from build123d import *

# Parameters (mm, degrees)
SKETCH_W        = 15.1
SKETCH_H        = 9
PAD_DEPTH       = 14.5
SKETCH001_W     = 13.1
SKETCH001_H     = 7
POCKET_DEPTH    = 13.5
SKETCH002_R     = 3.125
POCKET001_DEPTH = 5
POCKET002_DEPTH = 15.101


with BuildPart() as part:
    # Sketch → Pad (new body)
    with BuildSketch(Plane.XY):
        Rectangle(SKETCH_W, SKETCH_H)
    extrude(amount=PAD_DEPTH)

    # Sketch001 (on Face6 of Pad) → Pocket (cut)
    with BuildSketch(Plane.XY.offset(14.5)):
        Rectangle(SKETCH001_W, SKETCH001_H)
    extrude(amount=-POCKET_DEPTH, mode=Mode.SUBTRACT)

    # Sketch002 (on Face4 of Pocket) → Pocket001 (cut)
    with BuildSketch(Plane(origin=(0, 0, 0), x_dir=(1, 0, 0), z_dir=(0, 0, -1))):
        Circle(SKETCH002_R)
    extrude(amount=-POCKET001_DEPTH, mode=Mode.SUBTRACT)

    # Sketch003 (on Face2 of Pocket001) → Pocket002 (cut, through all)
    with BuildSketch(Plane(origin=(-7.55, 0, 0), x_dir=(0, -1, 0), z_dir=(-1, 0, 0))):
        with BuildLine():
            Line((-2.549494, 14.5), (2.549494, 14.5))
            Line((2.549494, 14.5), (2.549494, 11.50906))
            ThreePointArc((1.549494, 10.50906), (2.256601, 10.801953), (2.549494, 11.50906))
            Line((1.549494, 10.50906), (-1.549494, 10.50906))
            ThreePointArc((-2.549494, 11.50906), (-2.256601, 10.801953), (-1.549494, 10.50906))
            Line((-2.549494, 11.50906), (-2.549494, 14.5))
        make_face()
    extrude(amount=-POCKET002_DEPTH, mode=Mode.SUBTRACT)


solid = part.part
Geometry check sheet. Reference: the model listing, model coordinates, mm. A direction names the side the tool comes from. Coordinates: 2 decimals unless noted, no trailing zeros. Loops run counter-clockwise (first coordinate to the right, second up) from the corner with the lowest first, then second, coordinate; pieces in that order, holes last. Notation, with made-up numbers: (66.5, 70.25) - (99.5, 70.25) arc R24 ccw to (99.5, 84.25) - close; hole circle Ø4 at (-22, 69). An arc over 180 degrees is marked (long way). Use one line per item in the form item = value. Start each with the question number.
Item 1: Section check C-C, the plane z = 11.75. Enter the section's corners in (x, y).
Item 2: Thickness scan on probe 1 along Y at (x, z) = (0, 0.5) (3 decimals); probe 2 along Y at (x, z) = (-5, 12.5); probe 3 along X at (y, z) = (0.25, 4). Record the ranges inside material, lowest first.
Item 3: Section check D-D, the plane z = 7.75. Enter the section's corners in (x, y).
Item 4: Section check B-B, the plane y = 0. Enter the section's corners in (x, z) (3 decimals).
Item 5: Section check A-A, the plane x = 0. Enter the section's corners in (y, z) (3 decimals), and give its area (4 significant figures).
Item 6: Mould release check, pull along X, two halves, no side actions. Record for faces 1 (the face through (-6.55, 0, 6)), 2 (the face through (2.98, -0.94, 0.49)), 3 (the face through (7.55, 0, 7)), 4 (the face through (-3.5, 0.1, 0)): +X half, -X half, draft (parallel to the pull), parting line (faces both ways), or undercut.
Item 7: Gauge pin test, flat ends, axial feed: pin 1 (0.8 mm diameter, centred on x = 7, y = 0, fed in from +Z); pin 2 (2 mm diameter, centred on x = 2, y = 0.5, fed in from +Z). Record the tip position at first contact, or that the pin passes through.
Item 8: Tool access check on faces 5 (the face through (7, 0, 10.509)), 6 (the face through (-7.55, 0, 7)), 7 (the face through (6.55, 0, 6)). Record the directions out of +Z, -Z, +X, -X, +Y, -Y that give a thin tool (end or side, any length) a straight path to the whole face; none if there is none.
Computed:
q1.outline = (-7.55, -4.5) - (7.55, -4.5) - (7.55, -2.55) - (6.55, -2.55) - (6.55, -3.5) - (-6.55, -3.5) - (-6.55, -2.55) - (-7.55, -2.55) - close; (-7.55, 2.55) - (-6.55, 2.55) - (-6.55, 3.5) - (6.55, 3.5) - (6.55, 2.55) - (7.55, 2.55) - (7.55, 4.5) - (-7.55, 4.5) - close
q2.probe_1 = -4.5 to -3.125, 3.125 to 4.5
q2.probe_2 = -4.5 to -3.5, 3.5 to 4.5
q2.probe_3 = -7.55 to -6.55, 6.55 to 7.55
q3.outline = (-7.55, -4.5) - (7.55, -4.5) - (7.55, 4.5) - (-7.55, 4.5) - close; hole (-6.55, -3.5) - (6.55, -3.5) - (6.55, 3.5) - (-6.55, 3.5) - close
q4.outline = (-7.55, 0) - (-3.125, 0) - (-3.125, 1) - (-6.55, 1) - (-6.55, 10.509) - (-7.55, 10.509) - close; (3.125, 0) - (7.55, 0) - (7.55, 10.509) - (6.55, 10.509) - (6.55, 1) - (3.125, 1) - close
q5.outline = (-4.5, 0) - (-3.125, 0) - (-3.125, 1) - (-3.5, 1) - (-3.5, 14.5) - (-4.5, 14.5) - close; (3.125, 0) - (4.5, 0) - (4.5, 14.5) - (3.5, 14.5) - (3.5, 1) - (3.125, 1) - close
q5.area = 29.75 mm2
q6.face_1 = undercut
q6.face_2 = undercut
q6.face_3 = +X half
q6.face_4 = draft
q7.pin_1 = 10.51
q7.pin_2 = through
q8.face_5 = +Z, +X, -X
q8.face_6 = +Z, -Z, -X, +Y, -Y
q8.face_7 = +Z
